from build123d import *

# Parameters (mm, degrees)
F0_W     = 19.5
F0_H     = 10.6
F1_DEPTH = 6.3
F2_R     = 2.307824
F3_DEPTH = 25
F5_DEPTH = 25


with BuildPart() as f1:
    # F0 (on Front) → F1 (new body)
    with BuildSketch(Plane.XZ):
        with Locations((9.75, 5.3)):
            Rectangle(F0_W, F0_H)
    extrude(amount=F1_DEPTH)

    # F2 (on face) → F3 (cut)
    with BuildSketch(Plane.XZ.offset(6.3)):
        with Locations((5, 2.9)):
            Circle(F2_R)
        with Locations((14.5, 2.9)):
            Circle(F2_R)
    extrude(amount=-F3_DEPTH, mode=Mode.SUBTRACT)

    # F4 (on face) → F5 (cut)
    with BuildSketch(Plane.XZ.offset(6.3)):
        Polygon((10.5, 10.6), (0, 10.6), (0, 9.5), (9.2344, 9.5), align=None)
    extrude(amount=-F5_DEPTH, mode=Mode.SUBTRACT)


solid = f1.part
Geometry check sheet. Reference: the model listing, model coordinates, mm. A direction names the side the tool comes from. Round coordinates to 2 decimals unless told otherwise and drop trailing zeros. Write each loop counter-clockwise with the first axis right and the second up, starting at its lowest first coordinate (ties: lowest second). Pieces come first, ordered by that corner, then holes. Notation, with made-up numbers: (-36.5, 0.5) -> (-26.5, 0.5) arc R20 cw to (-26.5, 33.5) -> close; hole circle Ø2 at (55.5, -0.5). An arc over 180 degrees is marked (long way). One line per item, written item: value. Start each with the question number.
(1) Cross-section at B-B, the plane y = -1. Record the cut outline in (x, z), and give its area (3 significant figures).
(2) Go/stop test with a flat-tipped pin: pin 1 Ø1.9 at (x, y) = (5.5, -4) entering from +Z. Record where the tip stops, or that it passes through.
(3) Cross-section at C-C, the plane z = 2.9. Record the cut outline in (x, y), and give its area (3 significant figures).
(4) Draft check along X on faces 1 (the flat face through (0, -3, 5)), 2 (the cylindrical face through (3.3, -3.19, 4.46)), 3 (the flat face through (10, -3, 0)). Enter one of: +X half, -X half, draft (parallel to the pull), parting line (faces both ways), or undercut.
(5) Cross-section at D-D, the plane x = 14.5. Record the cut outline in (y, z).
(6) Access from +Z, -Z, +X, -X, +Y, -Y to the whole of each face (thin tool, end or side, straight path). Record for faces 4 (the flat face through (5, -3, 9.5)), 5 (the cylindrical face through (16.7, -3.2, 3.6)).
(7) Scan lines: line 1 (Z direction, x = 5, y = -3.75); line 2 (X direction, y = -1.75, z = 1.5); line 3 (Z direction, x = 14.5, y = -3). Record each from-to range of solid material in increasing order. Write a range as [from, to].
(8) Cross-section at A-A, the plane x = 5. Record the cut outline in (y, z), and give its area (3 significant figures).
Answer:
1. outline: (0, 0) -> (19.5, 0) -> (19.5, 10.6) -> (10.5, 10.6) -> (9.23, 9.5) -> (0, 9.5) -> close; hole circle Ø4.62 at (5, 2.9); hole circle Ø4.62 at (14.5, 2.9)
1. area: 162 mm²
2. pin 1: z = 9.5
3. outline: (0, -6.3) -> (2.69, -6.3) -> (2.69, 0) -> (0, 0) -> close; (7.31, -6.3) -> (12.19, -6.3) -> (12.19, 0) -> (7.31, 0) -> close; (16.81, -6.3) -> (19.5, -6.3) -> (19.5, 0) -> (16.81, 0) -> close
3. area: 64.7 mm²
4. face 1: -X half
4. face 2: undercut
4. face 3: draft
5. outline: (-6.3, 0) -> (0, 0) -> (0, 0.59) -> (-6.3, 0.59) -> close; (-6.3, 5.21) -> (0, 5.21) -> (0, 10.6) -> (-6.3, 10.6) -> close
6. face 4: +Z, -X, +Y, -Y
6. face 5: +Y, -Y
7. line 1: [0, 0.59], [5.21, 9.5]
7. line 2: [0, 3.17], [6.83, 12.67], [16.33, 19.5]
7. line 3: [0, 0.59], [5.21, 10.6]
8. outline: (-6.3, 0) -> (0, 0) -> (0, 0.59) -> (-6.3, 0.59) -> close; (-6.3, 5.21) -> (0, 5.21) -> (0, 9.5) -> (-6.3, 9.5) -> close
8. area: 30.8 mm²
